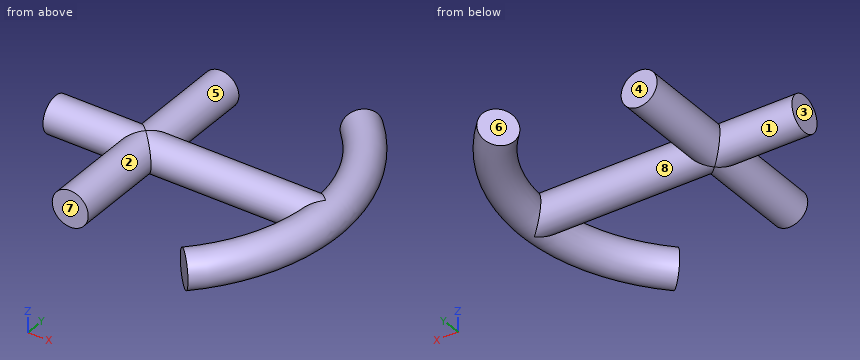
Autodesk Inventor part; units mm, degrees
ref_plane "Work Plane1" through (0, 76.2, 0) normal (0, 1, 0) x (1, 0, 0)
ref_plane "Work Plane3" through (139.7, 76.2, 12.7) normal (-1, 0, 0) x (0, 0, 1)
ref_plane "YZ Plane" through (0, 0, 0) normal (1, 0, 0) x (0, 1, 0)
sketch "Sketch1" plane through (0, 0, 0) normal (0, 1, 0) x (-1, 0, 0)
  circle A0 centre (0, 0) radius 12.7
  dimension "d0" = 25.4
extrude "Extrusion1" add sketch "Sketch1" along normal blind 152.4
sketch "Sketch2" plane through (0, 0, 0) normal (1, 0, 0) x (0, 1, 0)
  circle A0 centre (76.2, 0) radius 12.7
  point P0 (0, 0)
extrude "Extrusion2" add sketch "Sketch2" along normal blind 127 and the other way blind 63.5
ref_plane "Work Plane1" through (0, 76.2, 0) normal (0, 1, 0) x (1, 0, 0)
sketch "Sketch3" plane through (0, 76.2, 0) normal (0, 1, 0) x (1, 0, 0)
  line L0 (127, -12.7) -> (127, 12.7)
  circle A0 centre (127, 0) radius 12.7
  line L1 (0, -22.5547) -> (0, 28.0783)
  point P0 (0, 0)
revolve "Revolution1" add sketch "Sketch3" angle 90 mid plane about axis through (0, 76.2, 22.5547) along (0, 0, -1)
ref_plane "Work Plane3" through (139.7, 76.2, 12.7) normal (-1, 0, 0) x (0, 0, 1)
ref_plane "Work Plane2" through (127, 76.2, 12.7) normal (-1, 0, 0) x (0, 0, 1)
properties part number "anchorPlaceholder"
Design review of the part built by this model. Coordinates are the model's own, in mm. Face numbers are marked on the shaded views. A direction names the side the tool comes from. Round coordinates to 2 decimals unless told otherwise and drop trailing zeros. Write each loop counter-clockwise with the first axis right and the second up, starting at its lowest first coordinate (ties: lowest second). Pieces come first, ordered by that corner, then holes. Notation, with made-up numbers: (-25.5, 52.5) -> (-17.5, 52.5) arc R22 ccw to (-17.5, 74.5) -> close; hole circle Ø6 at (77.5, 56.25). An arc over 180 degrees is marked (long way). Answer in a Markdown table with one row per item.
Q1. Take a section at C-C, the plane x = 94. Count the separate pieces of the cut face and the enclosed holes in it, then the cut area to 3 significant figures.
The answers:
| item | result |
|---|---|
| separate pieces | 3 |
| enclosed holes | 0 |
| area | 1,730 mm² |
Q2. For the marked faces 1, 2, 3 and 4, list the 3-axis set-ups (+Z, -Z, +X, -X, +Y, -Y) from which the entire face can be reached by the end or side of a thin tool; tool diameter is ignored.
The answers:
| item | result |
|---|---|
| face 1 | -X |
| face 2 | -Y |
| face 3 | +Z, -Z, -X, +Y, -Y |
| face 4 | +Z, -Z, -X, +Y |
Q3. Take a section at A-A, the plane z = -7.75. State the section outline as (x, y) points.
The answers:
| item | result |
|---|---|
| outline | (-63.5, 66.14) -> (-10.06, 66.14) -> (-10.06, 0) -> (10.06, 0) -> (10.06, 66.14) -> (116.51, 66.14) arc R116.94 cw to (82.69, -6.49) -> (96.92, -20.72) arc R137.06 ccw to (96.92, 173.12) -> (82.69, 158.89) arc R116.94 cw to (116.51, 86.26) -> (10.06, 86.26) -> (10.06, 152.4) -> (-10.06, 152.4) -> (-10.06, 86.26) -> (-63.5, 86.26) -> close |
Q4. Clearance check with flat-ended pins moving along their axes: pin 1 Ø5 at (y, z) = (-1, 10) entering from -X; pin 2 Ø8 at (x, y) = (83.5, 77) entering from -Z; pin 3 Ø3 at (x, z) = (-24.5, 2.5) entering from +Y; pin 4 Ø12.5 at (x, z) = (3, 4.5) entering from -Y. State where each tip first meets the part, or that it passes through.
The answers:
| item | result |
|---|---|
| pin 1 | x = -10.09 |
| pin 2 | z = -12.7 |
| pin 3 | y = 88.86 |
| pin 4 | y = 0 |
Q5. Draft analysis for pull direction X (two halves, no side actions). For the marked faces 5, 6, 7 and 8, state which applies: +X half, -X half, draft (parallel to the pull), parting line (faces both ways), or undercut.
The answers:
| item | result |
|---|---|
| face 5 | undercut |
| face 6 | -X half |
| face 7 | draft |
| face 8 | undercut |
Q6. Take a section at D-D, the plane z = 9.75. State the section outline as (x, y) points, then the cut area to 3 significant figures.
The answers:
| item | result |
|---|---|
| outline | (-63.5, 68.06) -> (-8.14, 68.06) -> (-8.14, 0) -> (8.14, 0) -> (8.14, 68.06) -> (118.58, 68.06) arc R118.86 cw to (84.05, -7.85) -> (95.56, -19.36) arc R135.14 ccw to (95.56, 171.76) -> (84.05, 160.25) arc R118.86 cw to (118.58, 84.34) -> (8.14, 84.34) -> (8.14, 152.4) -> (-8.14, 152.4) -> (-8.14, 84.34) -> (-63.5, 84.34) -> close |
| area | 8,430 mm² |
Q7. Take a section at B-B, the plane x = 63.5. State the section outline as (y, z) points, then the cut area to 3 significant figures.
The answers:
| item | result |
|---|---|
| outline | circle Ø25.4 at (76.2, 0) |
| area | 507 mm² |
Q8. To check wall thickness, follow L1, parallel to Y at x = 97, z = 9; L2, parallel to Z at x = 128, y = 82; L3, parallel to X at y = 59, z = 4.75. State the ranges of each line that lie inside material, in increasing order. Write a range as [from, to].
The answers:
| item | result |
|---|---|
| L1 | [-19.07, 8.94], [67.24, 85.16], [143.46, 171.47] |
| L2 | [-12.65, 12.65] |
| L3 | [-11.78, 11.78], [113.93, 137.71] |
